```python
from build123d import *

# Parameters (mm, degrees)
SKETCH1_W           = 47
SKETCH1_H           = 23.6
SKETCH1_W_2         = 44.18
SKETCH1_H_2         = 19
BOSS_EXTRUDE1_DEPTH = 4.5
SKETCH6_W           = 7.25
SKETCH6_H           = 4.5
BOSS_EXTRUDE3_DEPTH = 5.25
SKETCH7_W           = 7.25
SKETCH7_H           = 4.5
BOSS_EXTRUDE4_DEPTH = 5.25
SKETCH8_R           = 1.5
CUT_EXTRUDE2_DEPTH  = 5.5
SKETCH10_W          = 1.41
SKETCH10_H          = 8
CUT_EXTRUDE3_DEPTH  = 1.5


with BuildPart() as part:
    # Sketch1 → Boss-Extrude1 (new body)
    with BuildSketch(Plane(origin=(0, 0, 0), x_dir=(1, 0, 0), z_dir=(0, 1, 0))):
        with Locations((22.09, 9.5)):
            Rectangle(SKETCH1_W, SKETCH1_H)
        with Locations((22.09, 9.5)):
            Rectangle(SKETCH1_W_2, SKETCH1_H_2, mode=Mode.SUBTRACT)
    extrude(amount=BOSS_EXTRUDE1_DEPTH)

    # Sketch6 → Boss-Extrude3 (add)
    with BuildSketch(Plane.XY.offset(2.3)):
        with Locations((2.215, 2.25)):
            Rectangle(SKETCH6_W, SKETCH6_H)
        with Locations((41.965, 2.25)):
            Rectangle(SKETCH6_W, SKETCH6_H)
    extrude(amount=BOSS_EXTRUDE3_DEPTH)

    # Sketch7 → Boss-Extrude4 (add)
    with BuildSketch(Plane(origin=(0, 0, -21.3), x_dir=(-1, 0, 0), z_dir=(0, 0, -1))):
        with Locations((-41.965, 2.25)):
            Rectangle(SKETCH7_W, SKETCH7_H)
        with Locations((-2.215, 2.25)):
            Rectangle(SKETCH7_W, SKETCH7_H)
    extrude(amount=BOSS_EXTRUDE4_DEPTH)

    # Sketch8 → Cut-Extrude2 (cut, through all)
    with BuildSketch(Plane(origin=(0, 4.5, 0), x_dir=(1, 0, 0), z_dir=(0, 1, 0))):
        with Locations((41.965, 22.925)):
            Circle(SKETCH8_R)
        with Locations((41.965, -3.925)):
            Circle(SKETCH8_R)
        with Locations((2.215, -3.925)):
            Circle(SKETCH8_R)
        with Locations((2.215, 22.925)):
            Circle(SKETCH8_R)
    extrude(amount=-CUT_EXTRUDE2_DEPTH, mode=Mode.SUBTRACT)

    # Sketch10 → Cut-Extrude3 (cut)
    with BuildSketch(Plane(origin=(0, 4.5, 0), x_dir=(1, 0, 0), z_dir=(0, 1, 0))):
        with Locations((-0.705, 9.5)):
            Rectangle(SKETCH10_W, SKETCH10_H)
    extrude(amount=-CUT_EXTRUDE3_DEPTH, mode=Mode.SUBTRACT)


solid = part.part
```
Could you check a few things on this model? Use its own coordinates, in mm. A direction names the side the tool comes from. Give positions to 0.01 mm unless a question says otherwise; leave off trailing zeros. Write each loop counter-clockwise with the first axis right and the second up, starting at its lowest first coordinate (ties: lowest second). Pieces come first, ordered by that corner, then holes. Notation, with made-up numbers: (59.5, -32.5) - (102.5, -32.5) arc R12 ccw to (102.5, -14.5) - close; hole circle Ø4 at (71.25, 55). An arc over 180 degrees is marked (long way). One line per item, written item: value. Start each with the question number.
Item 1: I'm going to push flat-ended pins straight in: pin 1 (2 mm diameter, centred on x = 21.5, y = 2.5, fed in from +Z); pin 2 (1 mm diameter, centred on x = 12.5, y = 2, fed in from -Z). Where does each tip first touch, or does it pass through?
Item 2: Imagine slicing it at A-A, the plane z = -11.5. List the corners of the cut face in (x, y) for me.
Item 3: Imagine slicing it at C-C, the plane y = 3.7. List the corners of the cut face in (x, z) for me (3 decimals).
Item 4: Imagine slicing it at B-B, the plane x = 25. List the corners of the cut face in (y, z) for me.
Item 5: If we mould it in two halves opening along Z, with no side actions, what happens to faces 1 (the face through (-1, 4, -13.5)), 2 (the face through (38.34, 2, 5)), 3 (the face through (2, 2, 7.55)), 4 (the face through (-1, 3, -10))? For each: +Z half, -Z half, draft (parallel to the pull), parting line (faces both ways), or undercut.
Item 6: Imagine slicing it at D-D, the plane y = 1.4. List the corners of the cut face in (x, z) for me (3 decimals).
Item 7: Please list where these lines run through material, in increasing order: line 1 (Z direction, x = 16, y = 4.1); line 2 (Z direction, x = 5.5, y = 1.8); line 3 (X direction, y = 2.2, z = -22). Write a range as from..to.
Item 8: Which directions (+Z, -Z, +X, -X, +Y, -Y) give clear straight access to the entire face, cutting with the end or side of a thin tool? Please do faces 5 (the face through (22, 2, 2.3)), 6 (the face through (42, 2, 7.55)), 7 (the face through (5.84, 2, -24)), 8 (the face through (44.18, 2, -9)), 9 (the face through (-1, 4, -5.5)).
Geometry says:
1. pin 1: z = 2.3
1. pin 2: z = -21.3
2. outline: (-1.41, 0) - (0, 0) - (0, 3) - (-1.41, 3) - close; (44.18, 0) - (45.59, 0) - (45.59, 4.5) - (44.18, 4.5) - close
3. outline: (-1.41, -26.55) - (5.84, -26.55) - (5.84, -21.3) - (38.34, -21.3) - (38.34, -26.55) - (45.59, -26.55) - (45.59, 7.55) - (38.34, 7.55) - (38.34, 2.3) - (5.84, 2.3) - (5.84, 7.55) - (-1.41, 7.55) - (-1.41, -5.5) - (0, -5.5) - (0, 0) - (44.18, 0) - (44.18, -19) - (0, -19) - (0, -13.5) - (-1.41, -13.5) - close; hole circle Ø3 at (2.215, -22.925); hole circle Ø3 at (2.215, 3.925); hole circle Ø3 at (41.965, -22.925); hole circle Ø3 at (41.965, 3.925)
4. outline: (0, -21.3) - (4.5, -21.3) - (4.5, -19) - (0, -19) - close; (0, 0) - (4.5, 0) - (4.5, 2.3) - (0, 2.3) - close
5. face 1: undercut
5. face 2: draft
5. face 3: +Z half
5. face 4: undercut
6. outline: (-1.41, -26.55) - (5.84, -26.55) - (5.84, -21.3) - (38.34, -21.3) - (38.34, -26.55) - (45.59, -26.55) - (45.59, 7.55) - (38.34, 7.55) - (38.34, 2.3) - (5.84, 2.3) - (5.84, 7.55) - (-1.41, 7.55) - close; hole (0, -19) - (44.18, -19) - (44.18, 0) - (0, 0) - close; hole circle Ø3 at (2.215, -22.925); hole circle Ø3 at (2.215, 3.925); hole circle Ø3 at (41.965, -22.925); hole circle Ø3 at (41.965, 3.925)
7. line 1: -21.3..-19, 0..2.3
7. line 2: -26.55..-19, 0..7.55
7. line 3: -1.41..1.03, 3.4..5.84, 38.34..40.78, 43.15..45.59
8. face 5: +Z, +Y, -Y
8. face 6: +Z, +X, -X, +Y, -Y
8. face 7: -Z, +Y, -Y
8. face 8: +Y, -Y
8. face 9: -X, +Y
